Part model, mm, in its own coordinate system. A direction names the side the tool comes from. Coordinates: 2 decimals unless noted, no trailing zeros. Write each loop counter-clockwise with the first axis right and the second up, starting at its lowest first coordinate (ties: lowest second). Pieces come first, ordered by that corner, then holes. Notation, with made-up numbers: (73, 32.25) -> (82, 32.25) arc R21 cw to (82, 56.25) -> close; hole circle Ø8 at (50.25, 77.5). An arc over 180 degrees is marked (long way). Write item = value, one per line. Start each with the question number.
Q1. Band-saw the part on A-A, the plane x = -25.5. List the corners of the cut face in (y, z).
Q2. Pull direction Y, two halves, no side cores. Call faces 4 (the flat face through (-95.56, -25.64, 24)), 5 (the cylindrical face through (-111.932, -25.56, 54.712)), 6 (the flat face through (-33, 0, 4)): released by +Y, released by -Y, zero draft, split by the parting line, or undercut.
Q3. Band-saw the part on B-B, the plane y = -13. List the corners of the cut face in (x, z).
Q4. Tool access for faces 1 (the cylindrical face through (-39.71, -25.78, -1.71)), 2 (the cylindrical face through (-117.922, -44.586, 60.306)), 3 (the flat face through (5, -14, 8.152)): list every direction of +Z, -Z, +X, -X, +Y, -Y with a clear straight run to the whole face (end or side of a thin tool).
Q5. Band-saw the part on C-C, the plane z = 17. List the corners of the cut face in (x, y), plus the area to 3 significant figures.
Q6. Probe line 1 (Z direction, x = 31, y = -40); line 2 (X direction, y = -20, z = 47.5); line 3 (X direction, y = -31, z = -2). List the from-to ranges inside material, lowest first.
Q7. Band-saw the part on D-D, the plane y = -38.5. List the corners of the cut face in (x, z).
Q8. Pin check, flat tips, straight feed: P1, Ø4, axis at x = -2, y = -44, coming from the +Z side; P2, Ø12, axis at y = -23, z = 21.5, coming from the +X side; P3, Ø1, axis at y = -42.5, z = 29, coming from the +X side; P4, Ø10, axis at x = -21, y = -24, coming from the +Z side. Stop position of each tip, or through.
from build123d import *

# Parameters (mm, degrees)
F1_DEPTH = 52
F2_R     = 10
F3_DEPTH = 20
F5_DEPTH = 20
F6_R     = 25.99999


# Not quite as in the source:
# - a fillet or chamfer is up to 0.001 mm smaller than in the source, because OpenCascade refuses the exact size


with BuildPart() as f1:
    # F0 (on Front) → F1 (new body)
    with BuildSketch(Plane.XZ):
        Polygon((60.2885049582, -11.8481526151), (60.2885049582, 8.1518473849), (-51.4272237944, 8.1518473849), (-116.2800375368, 73.0046611273), (-130.4221731605, 58.8625255035), (-59.7114950418, -11.8481526151), align=None)
    extrude(amount=F1_DEPTH)

    # F2 (on face) → F3 (cut)
    with BuildSketch(Plane(origin=(-21.6376882048, 0, -21.6376882048), x_dir=(0.7071067812, 0, -0.7071067812), z_dir=(0.7071067812, 0, 0.7071067812))):
        with Locations((-107.8444940002, -26)):
            Circle(F2_R)
    extrude(amount=-F3_DEPTH, mode=Mode.SUBTRACT)

    # F4 (on face) → F5 (cut)
    with BuildSketch(Plane.XY.offset(8.1518473849)):
        with BuildLine():
            ThreePointArc((40.2885049582, -36), (47.35957277, -33.0710678119), (50.2885049582, -26))
            ThreePointArc((50.2885049582, -26), (47.35957277, -18.9289321881), (40.2885049582, -16))
            ThreePointArc((40.2885049582, -16), (30.2885049582, -26), (40.2885049582, -36))
        make_face()
        with BuildLine():
            ThreePointArc((40.2885049582, -36), (30.2885049582, -26), (40.2885049582, -16))
            Line((40.2885049582, -16), (-29.7114950418, -16))
            ThreePointArc((-29.7114950418, -16), (-22.64042723, -18.9289321881), (-19.7114950418, -26))
            ThreePointArc((-19.7114950418, -26), (-22.64042723, -33.0710678119), (-29.7114950418, -36))
            Line((-29.7114950418, -36), (40.2885049582, -36))
        make_face()
        with BuildLine():
            ThreePointArc((-19.7114950418, -26), (-22.64042723, -18.9289321881), (-29.7114950418, -16))
            ThreePointArc((-29.7114950418, -16), (-39.7114950418, -26), (-29.7114950418, -36))
            ThreePointArc((-29.7114950418, -36), (-22.64042723, -33.0710678119), (-19.7114950418, -26))
        make_face()
    extrude(amount=-F5_DEPTH, mode=Mode.SUBTRACT)

    # F6 (radius 26 in the source; OpenCascade refuses exactly that, so slightly less here)
    f6_edges = [f1.edges().sort_by_distance(p)[0] for p in [
        (-123.351105, -52, 65.933593),
        (-123.351105, 0, 65.933593),
    ]]
    fillet(f6_edges, radius=F6_R)


solid = f1.part
Ans:
q1.outline = (-52, -11.85) -> (-36, -11.85) -> (-36, 8.15) -> (-52, 8.15) -> close; (-16, -11.85) -> (0, -11.85) -> (0, 8.15) -> (-16, 8.15) -> close
q2.face_4 = zero draft
q2.face_5 = undercut
q2.face_6 = released by +Y
q3.outline = (-127.96, 56.4) -> (-59.71, -11.85) -> (60.29, -11.85) -> (60.29, 8.15) -> (-51.43, 8.15) -> (-113.82, 70.54) -> close
q4.face_1 = +Z, -Z
q4.face_2 = +Z, -X, -Y
q4.face_3 = +Z, +X, +Y, -Y
q5.outline = (-88.56, -52) -> (-60.28, -52) -> (-60.28, 0) -> (-88.56, 0) -> close
q5.area = 1,470 mm2
q6.line_1 = -11.85 to 8.15
q6.line_2 = -119.06 to -116.33, -93.7 to -90.78
q6.line_3 = -69.56 to -38.37, 48.95 to 60.29
q7.outline = (-128.16, 56.6) -> (-59.71, -11.85) -> (60.29, -11.85) -> (60.29, 8.15) -> (-51.43, 8.15) -> (-114.02, 70.74) -> close
q8.P1 = 8.15
q8.P2 = -58.78
q8.P3 = -71.78
q8.P4 = through
